Can you work these out from the model? Positions are in its coordinate system, mm. Face numbers are marked on the shaded views. A direction names the side the tool comes from. Coordinates: 2 decimals unless noted, no trailing zeros. Loops run counter-clockwise (first coordinate to the right, second up) from the corner with the lowest first, then second, coordinate; pieces in that order, holes last. Notation, with made-up numbers: M 12.25,41.5 L 50.25,41.5 A31 ccw 50.25,70.5 Z; hole C 50.5,23 d8. An arc over 180 degrees is marked long. Return JSON: item names as keys, results as strings. Group by question number.
```python
from build123d import *

# Parameters (mm, degrees)
F0_W     = 42.6243245602
F0_H     = 17.7194328527
F2_W     = 13.1365954876
F2_H     = 19.5219665766
F3_DEPTH = 78.1549476087


with BuildPart() as f1:
    # F0 (on Front) → F1 (revolve)
    with BuildSketch(Plane.XZ):
        with Locations((21.3121622801, 28.1459019294)):
            Rectangle(F0_W, F0_H)
    revolve(axis=Axis((9.0612024069, 0, 0), (1, 0, 0)))

    # F2 (on Right) → F3 (cut)
    with BuildSketch(Plane.YZ):
        with Locations((0, 15.3909772635)):
            Rectangle(F2_W, F2_H)
    extrude(amount=F3_DEPTH, mode=Mode.SUBTRACT)


solid = f1.part
```
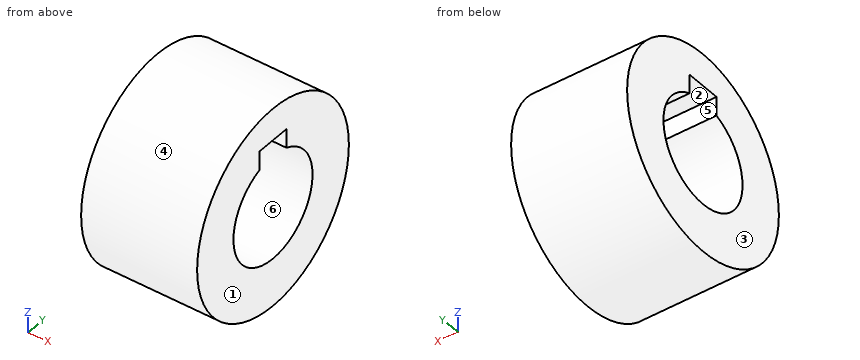
1) Suppose I cut it at D-D, the plane z = -23. List the corners of the cut face in (x, y) for me, then the cut area to 3 significant figures.
2) Suppose I cut it at B-B, the plane y = 12. List the corners of the cut face in (x, z) for me.
3) If I drill on line 1 (Y direction, x = 11, z = 0); line 2 (Z direction, x = 32, y = 0); line 3 (Y direction, x = 11, z = 9), over which ranges is the centre line in solid material (lowest first)? Write a range as from..to.
4) Suppose I cut it at A-A, the plane z = 0. List the corners of the cut face in (x, y) for me.
5) If we mould it in two halves opening along Z, with no side actions, what happens to the marked faces 3, 4, 5 and 6? For each: +Z half, -Z half, draft (parallel to the pull), parting line (faces both ways), or undercut.
6) For the marked faces 1 and 2, which set-ups out of +Z, -Z, +X, -X, +Y, -Y let a thin tool reach every point of the face, with its end or its side?
7) For pin 1 (3 mm diameter, centred on x = 26.5, z = 15.5, fed in from -Y); pin 2 (1 mm diameter, centred on y = 17, z = 28.5, fed in from -X); pin 3 (1.5 mm diameter, centred on x = 36.5, y = 9.5, fed in from -Z); pin 4 (1 mm diameter, centred on x = 25.5, y = 24.5, fed in from -Z), each with a flat end and sliding along its axis, tell me the tip position at first contact or that it passes through.
8) Suppose I cut it at C-C, the plane x = 3. List the corners of the cut face in (y, z) for me, then the cut area to 3 significant figures.
Returned:
{
 "1": {"outline": "M 0,-28.99 L 42.62,-28.99 L 42.62,28.99 L 0,28.99 Z", "area": "2,470 mm²"},
 "2": {"outline": "M 0,-35.01 L 42.62,-35.01 L 42.62,-15.1 L 0,-15.1 Z; M 0,15.1 L 42.62,15.1 L 42.62,35.01 L 0,35.01 Z"},
 "3": {"line 1": "y = -37.01..-19.29, 19.29..37.01", "line 2": "z = -37.01..-19.29, 25.15..37.01", "line 3": "y = -35.89..-17.06, 17.06..35.89"},
 "4": {"outline": "M 0,-37.01 L 42.62,-37.01 L 42.62,-19.29 L 0,-19.29 Z; M 0,19.29 L 42.62,19.29 L 42.62,37.01 L 0,37.01 Z"},
 "5": {"face 3": "draft", "face 4": "parting line", "face 5": "undercut", "face 6": "undercut"},
 "6": {"face 1": "+Z, -Z, +X, +Y, -Y", "face 2": "+X, -X"},
 "7": {"pin 1": "stops at y = -34.26", "pin 2": "stops at x = 0", "pin 3": "stops at z = -35.96", "pin 4": "stops at z = -28.17"},
 "8": {"outline": "C 0,0 d74.01; hole M -6.57,18.13 A19.29 ccw long 6.57,18.13 L 6.57,25.15 L -6.57,25.15 Z", "area": "3,050 mm²"}
}
